```python
from build123d import *

# Parameters (mm, degrees)
BOSS_EXTRUDE1_DEPTH = 25
EXTRUDE_THIN2_DEPTH = 5
SKETCH3_R           = 5
SKETCH3_R_2         = 3.75
SKETCH3_R_3         = 2.5
CUT_EXTRUDE1_DEPTH  = 1
SKETCH4_R           = 5
SKETCH4_R_2         = 1.25
SKETCH4_R_3         = 4
SKETCH4_R_4         = 2.75
SKETCH4_R_5         = 1.5
BOSS_EXTRUDE2_DEPTH = 1
SKETCH5_R           = 9.5
BOSS_EXTRUDE4_DEPTH = 20
BOSS_EXTRUDE5_START = 20
SKETCH7_R           = 9.5
BOSS_EXTRUDE5_DEPTH = 20


with BuildPart() as part:
    # Sketch1 → Boss-Extrude1 (new body)
    with BuildSketch(Plane.XY):
        with BuildLine():
            Line((-48.13609402, 12.5), (48.13609402, 12.5))
            ThreePointArc((48.13609402, 12.5), (60.63609402, 0), (48.13609402, -12.5))
            Line((48.13609402, -12.5), (-48.13609402, -12.5))
            ThreePointArc((-48.13609402, -12.5), (-60.63609402, 0), (-48.13609402, 12.5))
        make_face()
    extrude(amount=BOSS_EXTRUDE1_DEPTH)

    # Sketch2 → Extrude-Thin2 (add)
    with BuildSketch(Plane.XY.offset(25)):
        with BuildLine():
            Line((48.13609402, -12.5), (-48.13609402, -12.5))
            ThreePointArc((-48.13609402, -12.5), (-60.63609402, 0), (-48.13609402, 12.5))
            Line((-48.13609402, 12.5), (48.13609402, 12.5))
            ThreePointArc((48.13609402, 12.5), (60.63609402, 0), (48.13609402, -12.5))
        make_face()
        with BuildLine():
            Line((48.13609402, -7.5), (-48.13609402, -7.5))
            ThreePointArc((-48.13609402, -7.5), (-55.63609402, 0), (-48.13609402, 7.5))
            Line((-48.13609402, 7.5), (48.13609402, 7.5))
            ThreePointArc((48.13609402, 7.5), (55.63609402, 0), (48.13609402, -7.5))
        make_face(mode=Mode.SUBTRACT)
    extrude(amount=EXTRUDE_THIN2_DEPTH)

    # Sketch3 → Cut-Extrude1 (cut)
    with BuildSketch(Plane.XY.offset(25)):
        with Locations((-40, 0)):
            Circle(SKETCH3_R)
        with Locations((25, 0)):
            Circle(SKETCH3_R_2)
        with Locations((45, 0)):
            Circle(SKETCH3_R_3)
        with BuildLine():
            Line((-10, 6), (5, 6))
            ThreePointArc((5, 6), (11, 0), (5, -6))
            Line((5, -6), (-10, -6))
            ThreePointArc((-10, -6), (-16, 0), (-10, 6))
        make_face()
    extrude(amount=-CUT_EXTRUDE1_DEPTH, mode=Mode.SUBTRACT)

    # Sketch4 → Boss-Extrude2 (add)
    with BuildSketch(Plane.XY.offset(24)):
        with Locations((-5, 0)):
            Circle(SKETCH4_R)
        with Locations((5, 0)):
            Circle(SKETCH4_R_2)
        with Locations((-40, 0)):
            Circle(SKETCH4_R_3)
        with Locations((25, 0)):
            Circle(SKETCH4_R_4)
        with Locations((45, 0)):
            Circle(SKETCH4_R_5)
    extrude(amount=BOSS_EXTRUDE2_DEPTH)

    # Sketch5 → Boss-Extrude4 (add)
    with BuildSketch(Plane(origin=(0, 12.5, 0), x_dir=(1, 0, 0), z_dir=(0, 1, 0))):
        with Locations(Location((0, -15, 0), (0, 0, 90))):
            Circle(SKETCH5_R)
    extrude(amount=BOSS_EXTRUDE4_DEPTH)

    # Sketch7 → Boss-Extrude5 (add)
    with BuildSketch(Plane.XZ.offset(12.5).offset(BOSS_EXTRUDE5_START)):
        with Locations(Location((0, 15, 0), (0, 0, 270))):
            Circle(SKETCH7_R)
    extrude(amount=-BOSS_EXTRUDE5_DEPTH)


solid = part.part
```
Here's how the part is built. I have some questions about the finished solid (model axes, mm). A direction names the side the tool comes from. Round coordinates to 2 decimals unless told otherwise and drop trailing zeros. Write each loop counter-clockwise with the first axis right and the second up, starting at its lowest first coordinate (ties: lowest second). Pieces come first, ordered by that corner, then holes.
Q1. If we section it at D-D on y = -14.5: Write out the boundary of the cut face in (x, z).
Q2. Please list where these lines run through material, in increasing order: probe 1 along Y at (x, z) = (45, 24.7); probe 2 along Y at (x, z) = (25, 24.25); probe 3 along Y at (x, z) = (-21, 2).
Q3. If we section it at B-B on x = -40: Write out the boundary of the cut face in (y, z).
Q4. Which directions (+Z, -Z, +X, -X, +Y, -Y) give clear straight access to the entire face, cutting with the end or side of a thin tool? Please do faces 1 (the cylindrical face through (-60.633, -0.275, 14.79)), 2 (the flat face through (24, 3, 24)).
Q5. If we mould it in two halves opening along Y, with no side actions, what happens to faces 3 (the cylindrical face through (9.274, 22.36, 17.059)), 4 (the flat face through (45, 0, 25)), 5 (the flat face through (0, -32.5, 15))? For each: +Y half, -Y half, draft (parallel to the pull), parting line (faces both ways), or undercut.
Q6. If we section it at A-A on z = 27.25: Write out the boundary of the cut face in (x, y).
Q7. If we section it at C-C on z = 15: Write out the boundary of the cut face in (x, y), plus the area to 3 significant figures.
Q8. Will these pins go through, and if not, where does the flat tip stop? P1, Ø3, axis at x = 24, y = 0.5, coming from the +Z side; P2, Ø0.5, axis at x = -3.5, z = 24.5, coming from the +Y side; P3, Ø3, axis at y = 22.5, z = 13.5, coming from the +X side; P4, Ø4, axis at x = -24, y = -15, coming from the +Z side.
Answer below:
1. outline: circle Ø19 at (0, 15)
2. probe 1: y = -12.5 to -2.5, -1.5 to 1.5, 2.5 to 12.5
2. probe 2: y = -12.5 to -3.75, -2.75 to 2.75, 3.75 to 12.5
2. probe 3: y = -12.5 to 12.5
3. outline: (-12.5, 0) - (12.5, 0) - (12.5, 30) - (7.5, 30) - (7.5, 25) - (5, 25) - (5, 24) - (4, 24) - (4, 25) - (-4, 25) - (-4, 24) - (-5, 24) - (-5, 25) - (-7.5, 25) - (-7.5, 30) - (-12.5, 30) - close
4. face 1: +Z, -Z, -X
4. face 2: +Z
5. face 3: draft
5. face 4: undercut
5. face 5: -Y half
6. outline: (-48.14, -12.5) - (48.14, -12.5) arc R12.5 ccw to (48.14, 12.5) - (-48.14, 12.5) arc R12.5 ccw to start; hole (-48.14, -7.5) - (48.14, -7.5) arc R7.5 ccw to (48.14, 7.5) - (-48.14, 7.5) arc R7.5 ccw to start
7. outline: (-48.14, -12.5) - (-9.5, -12.5) - (-9.5, -32.5) - (9.5, -32.5) - (9.5, -12.5) - (48.14, -12.5) arc R12.5 ccw to (48.14, 12.5) - (9.5, 12.5) - (9.5, 32.5) - (-9.5, 32.5) - (-9.5, 12.5) - (-48.14, 12.5) arc R12.5 ccw to start
7. area: 3,660 mm2
8. P1: stops at z = 25
8. P2: stops at y = 12.5
8. P3: stops at x = 9.5
8. P4: passes through
